Source: CAD feature listing. Evaluate the final solid. Frame: model axes, mm. Face numbers are marked on the shaded views. Coordinates: 2 decimals unless noted, no trailing zeros. Order: outer loops, then holes, each group sorted by start corner. A loop starts at its lowest first (then second) coordinate and runs counter-clockwise, first axis right, second up. Notation, with made-up numbers: (75.25, 1) -> (88.25, 1) arc R28 cw to (88.25, 22) -> close; hole circle Ø6 at (89.25, 62). An arc over 180 degrees is marked (long way). Put each result on its own line as item: value.
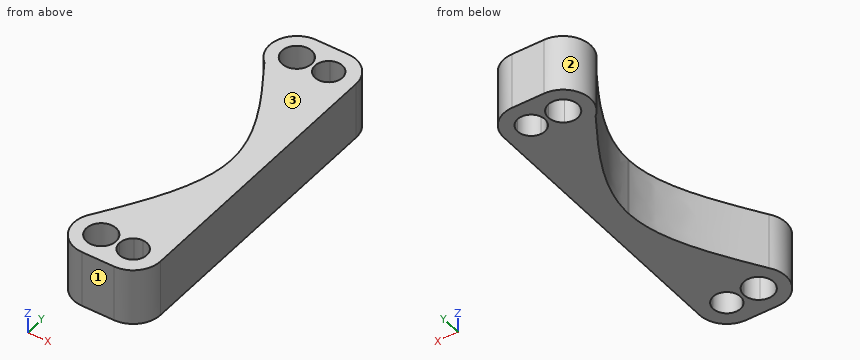
from build123d import *

# Parameters (mm, degrees)
F1_DEPTH = 25


with BuildPart() as f1:
    # F0 (on Top) → F1 (new body)
    with BuildSketch(Plane.XY):
        with BuildLine():
            ThreePointArc((-37.4794265696, 66.11101252), (-31.4088692079, 66.2372293657), (-28.3365694268, 61))
            ThreePointArc((-28.3365694268, 61), (-30.0939287397, 56.7573593129), (-34.3365694268, 55))
            Line((-34.3365694268, 55), (-34.3365694268, 49))
            ThreePointArc((-34.3365694268, 49), (-25.8512880525, 52.5147186258), (-22.3365694268, 61))
            ThreePointArc((-22.3365694268, 61), (-25.8512880525, 69.4852813742), (-34.3365694268, 73))
            ThreePointArc((-34.3365694268, 73), (-38.0134205158, 72.4228177815), (-41.3365694268, 70.7467943448))
            ThreePointArc((-41.3365694268, 70.7467943448), (-39.1120365911, 68.6751543283), (-37.4794265696, 66.11101252))
        make_face()
        with BuildLine():
            ThreePointArc((-48.3365694268, 73), (-44.6597183377, 72.4228177815), (-41.3365694268, 70.7467943448))
            ThreePointArc((-41.3365694268, 70.7467943448), (-38.0134205158, 72.4228177815), (-34.3365694268, 73))
            Line((-34.3365694268, 73), (-48.3365694268, 73))
        make_face()
        with BuildLine():
            ThreePointArc((-44.9704979982, 66.5605362275), (-43.3985807086, 68.8663810948), (-41.3365694268, 70.7467943448))
            ThreePointArc((-41.3365694268, 70.7467943448), (-44.6597183377, 72.4228177815), (-48.3365694268, 73))
            ThreePointArc((-48.3365694268, 73), (-59.5808573116, 65.1911800205), (-56.1910418813, 51.927664994))
            ThreePointArc((-56.1910418813, 51.927664994), (-48.8808622191, 49.0123502989), (-41.3365694268, 51.2532056552))
            ThreePointArc((-41.3365694268, 51.2532056552), (-43.3985807086, 53.1336189052), (-44.9704979982, 55.4394637725))
            ThreePointArc((-44.9704979982, 55.4394637725), (-54.8365694268, 61), (-44.9704979982, 66.5605362275))
        make_face()
        with BuildLine():
            ThreePointArc((-22.3365694268, 61), (-25.8512880525, 52.5147186258), (-34.3365694268, 49))
            Line((-34.3365694268, 49), (-34.3365694268, 0.6114759034))
            add(Edge.make_bspline(
                [(-34.3365694268, 0.6114759034), (-34.3350602132, 0.4076747809), (-34.3350542847, 0.2038495718), (-34.3365694268, 0)],
                knots=[0.4891390328, 0.4891390328, 0.4891390328, 0.4891390328, 0.4949274413, 0.4949274413, 0.4949274413, 0.4949274413], degree=3))
            Line((-34.3365694268, 0), (-34.3365694268, -49))
            ThreePointArc((-34.3365694268, -49), (-25.8512880525, -52.5147186258), (-22.3365694268, -61))
            Line((-22.3365694268, -61), (-22.3365694268, 61))
        make_face()
        with BuildLine():
            Line((-34.3365694268, 0.6114759034), (-34.3365694268, 49))
            ThreePointArc((-34.3365694268, 49), (-38.0134205158, 49.5771822185), (-41.3365694268, 51.2532056552))
            ThreePointArc((-41.3365694268, 51.2532056552), (-48.8808622191, 49.0123502989), (-56.1910418813, 51.927664994))
            add(Edge.make_bspline(
                [(-56.1910418813, 51.927664994), (-45.3262801206, 34.8831717712), (-34.4641028, 17.8333225018), (-34.3365694268, 0.6114759034)],
                knots=[0, 0, 0, 0, 0.4891390328, 0.4891390328, 0.4891390328, 0.4891390328], degree=3))
        make_face()
        with BuildLine():
            add(Edge.make_bspline(
                [(-34.3365694268, 0.6114759034), (-34.3350602132, 0.4076747809), (-34.3350542847, 0.2038495718), (-34.3365694268, 0)],
                knots=[0.4891390328, 0.4891390328, 0.4891390328, 0.4891390328, 0.4949274413, 0.4949274413, 0.4949274413, 0.4949274413], degree=3))
            Line((-34.3365694268, 0.6114759034), (-34.3365694268, 0))
        make_face()
        with BuildLine():
            Line((-34.3365694268, -49), (-34.3365694268, 0))
            add(Edge.make_bspline(
                [(-34.3365694268, 0), (-34.4687744467, -17.7870694727), (-46.1817789108, -35.7596268619), (-57.889438977, -53.7375841928)],
                knots=[0.4949274413, 0.4949274413, 0.4949274413, 0.4949274413, 1, 1, 1, 1], degree=3))
            ThreePointArc((-57.889438977, -53.7375841928), (-50.1176701861, -49.1329161086), (-41.3365694268, -51.2532056552))
            ThreePointArc((-41.3365694268, -51.2532056552), (-38.0134205158, -49.5771822185), (-34.3365694268, -49))
        make_face()
        with BuildLine():
            ThreePointArc((-34.3365694268, -73), (-25.8512880525, -69.4852813742), (-22.3365694268, -61))
            ThreePointArc((-22.3365694268, -61), (-25.8512880525, -52.5147186258), (-34.3365694268, -49))
            Line((-34.3365694268, -49), (-34.3365694268, -55))
            ThreePointArc((-34.3365694268, -55), (-30.0939287397, -56.7573593129), (-28.3365694268, -61))
            ThreePointArc((-28.3365694268, -61), (-31.4088692079, -66.2372293657), (-37.4794265696, -66.11101252))
            ThreePointArc((-37.4794265696, -66.11101252), (-39.1120365911, -68.6751543283), (-41.3365694268, -70.7467943448))
            ThreePointArc((-41.3365694268, -70.7467943448), (-38.0134205158, -72.4228177815), (-34.3365694268, -73))
        make_face()
        with BuildLine():
            ThreePointArc((-41.3365694268, -51.2532056552), (-50.1176701861, -49.1329161086), (-57.889438977, -53.7375841928))
            ThreePointArc((-57.889438977, -53.7375841928), (-59.087127312, -66.3315574795), (-48.3365694268, -73))
            ThreePointArc((-48.3365694268, -73), (-44.6597183377, -72.4228177815), (-41.3365694268, -70.7467943448))
            ThreePointArc((-41.3365694268, -70.7467943448), (-43.3985807086, -68.8663810948), (-44.9704979982, -66.5605362275))
            ThreePointArc((-44.9704979982, -66.5605362275), (-54.8365694268, -61), (-44.9704979982, -55.4394637725))
            ThreePointArc((-44.9704979982, -55.4394637725), (-43.3985807086, -53.1336189052), (-41.3365694268, -51.2532056552))
        make_face()
        with BuildLine():
            Line((-48.3365694268, -73), (-34.3365694268, -73))
            ThreePointArc((-34.3365694268, -73), (-38.0134205158, -72.4228177815), (-41.3365694268, -70.7467943448))
            ThreePointArc((-41.3365694268, -70.7467943448), (-44.6597183377, -72.4228177815), (-48.3365694268, -73))
        make_face()
        with BuildLine():
            ThreePointArc((-37.4794265696, 55.88898748), (-39.5737987924, 58.0722997812), (-40.3365694268, 61))
            Line((-40.3365694268, 61), (-41.8365694268, 61))
            ThreePointArc((-41.8365694268, 61), (-42.6739965007, 57.8085633553), (-44.9704979982, 55.4394637725))
            ThreePointArc((-44.9704979982, 55.4394637725), (-43.3985807086, 53.1336189052), (-41.3365694268, 51.2532056552))
            ThreePointArc((-41.3365694268, 51.2532056552), (-39.1120365911, 53.3248456717), (-37.4794265696, 55.88898748))
        make_face()
        with BuildLine():
            ThreePointArc((-40.3365694268, 61), (-39.5737987924, 63.9277002188), (-37.4794265696, 66.11101252))
            ThreePointArc((-37.4794265696, 66.11101252), (-39.1120365911, 68.6751543283), (-41.3365694268, 70.7467943448))
            ThreePointArc((-41.3365694268, 70.7467943448), (-43.3985807086, 68.8663810948), (-44.9704979982, 66.5605362275))
            ThreePointArc((-44.9704979982, 66.5605362275), (-42.6739965007, 64.1914366447), (-41.8365694268, 61))
            Line((-41.8365694268, 61), (-40.3365694268, 61))
        make_face()
        with BuildLine():
            Line((-34.3365694268, 49), (-34.3365694268, 55))
            ThreePointArc((-34.3365694268, 55), (-35.9696531478, 55.2265229229), (-37.4794265696, 55.88898748))
            ThreePointArc((-37.4794265696, 55.88898748), (-39.1120365911, 53.3248456717), (-41.3365694268, 51.2532056552))
            ThreePointArc((-41.3365694268, 51.2532056552), (-38.0134205158, 49.5771822185), (-34.3365694268, 49))
        make_face()
        with BuildLine():
            Line((-34.3365694268, -55), (-34.3365694268, -49))
            ThreePointArc((-34.3365694268, -49), (-38.0134205158, -49.5771822185), (-41.3365694268, -51.2532056552))
            ThreePointArc((-41.3365694268, -51.2532056552), (-39.1120365911, -53.3248456717), (-37.4794265696, -55.88898748))
            ThreePointArc((-37.4794265696, -55.88898748), (-35.9696531478, -55.2265229229), (-34.3365694268, -55))
        make_face()
        with BuildLine():
            ThreePointArc((-37.4794265696, -55.88898748), (-39.1120365911, -53.3248456717), (-41.3365694268, -51.2532056552))
            ThreePointArc((-41.3365694268, -51.2532056552), (-43.3985807086, -53.1336189052), (-44.9704979982, -55.4394637725))
            ThreePointArc((-44.9704979982, -55.4394637725), (-42.6739965007, -57.8085633553), (-41.8365694268, -61))
            Line((-41.8365694268, -61), (-40.3365694268, -61))
            ThreePointArc((-40.3365694268, -61), (-39.5737987924, -58.0722997812), (-37.4794265696, -55.88898748))
        make_face()
        with BuildLine():
            ThreePointArc((-44.9704979982, -66.5605362275), (-43.3985807086, -68.8663810948), (-41.3365694268, -70.7467943448))
            ThreePointArc((-41.3365694268, -70.7467943448), (-39.1120365911, -68.6751543283), (-37.4794265696, -66.11101252))
            ThreePointArc((-37.4794265696, -66.11101252), (-39.5737987924, -63.9277002188), (-40.3365694268, -61))
            Line((-40.3365694268, -61), (-41.8365694268, -61))
            ThreePointArc((-41.8365694268, -61), (-42.6739965007, -64.1914366447), (-44.9704979982, -66.5605362275))
        make_face()
    extrude(amount=F1_DEPTH)


solid = f1.part
1. First-contact query: pin 1 (2 mm diameter, centred on y = 42.5, z = 10.5, fed in from -X); pin 2 (0.5 mm diameter, centred on y = 0.5, z = 11.5, fed in from -X); pin 3 (3 mm diameter, centred on y = 25.5, z = 19.5, fed in from -X). Flat tips, straight axial feed; report the tip coordinate or a pass-through.
Numbers:
pin 1: stops at x = -50.87
pin 2: stops at x = -34.34
pin 3: stops at x = -41.56
2. Cut plane A-A on x = -31. Output: boundary loops of the cut face in (y, z).
Numbers:
outline: (-72.53, 0) -> (-65.99, 0) -> (-65.99, 25) -> (-72.53, 25) -> close; (-56.01, 0) -> (56.01, 0) -> (56.01, 25) -> (-56.01, 25) -> close; (65.99, 0) -> (72.53, 0) -> (72.53, 25) -> (65.99, 25) -> close
3. Ray query, line 1 along X through (y, z) = (-61, 9.5); line 2 along Y through (x, z) = (-52.5, 3.25); line 3 along Y through (x, z) = (-49, 5.25). Return the intervals inside material, ascending.
Numbers:
line 1: x = -60.34 to -54.84, -41.84 to -40.34, -28.34 to -22.34
line 2: y = -72.25 to -65.99, -56.01 to -45.4, 46.11 to 56.01, 65.99 to 72.25
line 3: y = -72.98 to -67.47, -54.53 to -39.78, 40.45 to 54.53, 67.47 to 72.98
4. Cut plane B-B on z = 13.25. Count the separate pieces of the cut face and the enclosed holes in it, plus the area to 3 significant figures.
Numbers:
separate pieces: 1
enclosed holes: 4
area: 3,070 mm2
5. Pull-direction query (Y, two-part tool) for the marked faces 1, 2 and 3; classes: pulls with the +Y half, pulls with the -Y half, needs draft (parallel to the pull), parting line crosses it, or undercut.
Numbers:
face 1: pulls with the -Y half
face 2: undercut
face 3: needs draft
